Could you check a few things on this drawing? It's one solid part, dimensions in mm from its lowest x, y, z. Coordinates: 2 decimals unless noted, no trailing zeros. Order: outer loops, then holes, each group sorted by start corner. A loop starts at its lowest first (then second) coordinate and runs counter-clockwise, first axis right, second up.
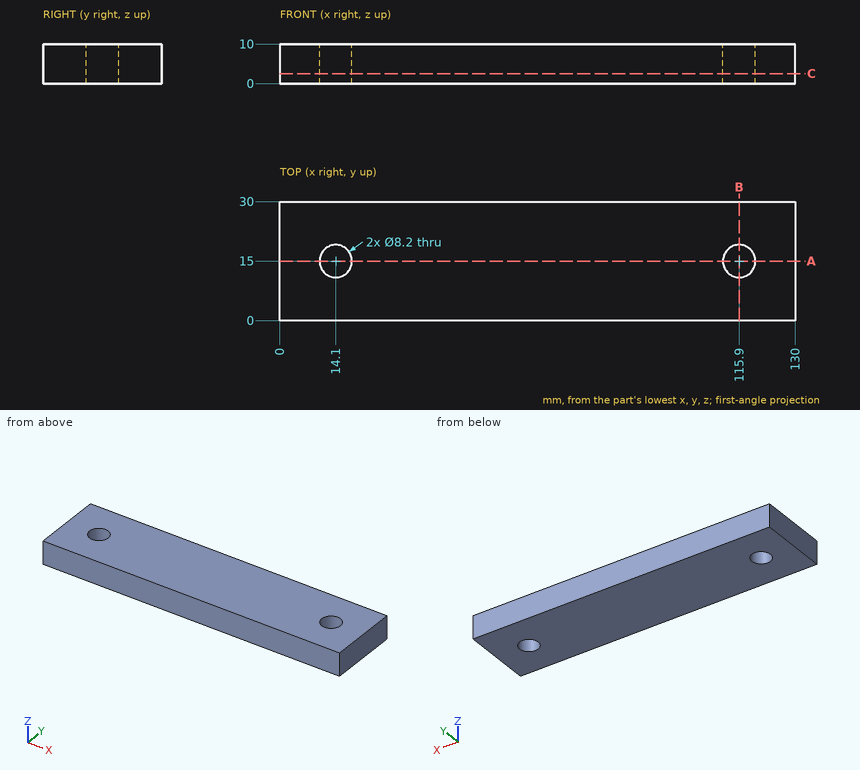
Q1. If we section it at C-C on z = 2.5: Write out the boundary of the cut face in (x, y), then the cut area to 3 significant figures.
Q2. If we section it at A-A on y = 15: Write out the boundary of the cut face in (x, z).
Q3. I need wall thicknesses on L1, parallel to X at y = 15, z = 3; L2, parallel to X at y = 13, z = 4.25; L3, parallel to Y at x = 115.9, z = 7.75. Which ranges of each line are inside material? Lowest first, please.
Q4. If we section it at B-B on x = 115.9: Write out the boundary of the cut face in (y, z), then the cut area to 3 significant figures.
Q5. Will this pin go through, and if not, where does the flat tip stop? pin 1 (5 mm diameter, centred on x = 14.1, y = 15, fed in from -Z).
Reply:
1. outline: (0, 0) - (130, 0) - (130, 30) - (0, 30) - close; hole circle Ø8.2 at (14.1, 15); hole circle Ø8.2 at (115.9, 15)
1. area: 3,790 mm2
2. outline: (0, 0) - (10, 0) - (10, 10) - (0, 10) - close; (18.2, 0) - (111.8, 0) - (111.8, 10) - (18.2, 10) - close; (120, 0) - (130, 0) - (130, 10) - (120, 10) - close
3. L1: x = 0 to 10, 18.2 to 111.8, 120 to 130
3. L2: x = 0 to 10.52, 17.68 to 112.32, 119.48 to 130
3. L3: y = 0 to 10.9, 19.1 to 30
4. outline: (0, 0) - (10.9, 0) - (10.9, 10) - (0, 10) - close; (19.1, 0) - (30, 0) - (30, 10) - (19.1, 10) - close
4. area: 218 mm2
5. pin 1: passes through
